Work out the finished part from the listing and answer in its coordinate system (mm). A direction names the side the tool comes from. Give positions to 0.01 mm unless a question says otherwise; leave off trailing zeros. Loops run counter-clockwise (first coordinate to the right, second up) from the corner with the lowest first, then second, coordinate; pieces in that order, holes last. Notation, with made-up numbers: (71.25, 34.25) - (122.25, 34.25) arc R31 cw to (122.25, 67.25) - close; hole circle Ø4 at (27.5, 13). An arc over 180 degrees is marked (long way). One line per item, written item: value.
from build123d import *

# Parameters (mm, degrees)
F1_DEPTH  = 15
F4_DEPTH  = 80
F6_DEPTH  = 80
F7_DEPTH  = 80
F9_DEPTH  = 30
F11_D     = 15
F11_DEPTH = 80
F11_TIP   = 4.5064546427
F14_D     = 15
F14_DEPTH = 80
F14_TIP   = 4.5064546427
F15_D     = 15
F15_DEPTH = 80
F15_TIP   = 4.5064546427


with BuildPart() as f1:
    # F0 (on Top) → F1 (new body)
    with BuildSketch(Plane.XY):
        Polygon((-20, 0), (0, 0), (20, 0), (40, 34.6410161514), (20, 69.2820323028), (0, 69.2820323028), (-20, 69.2820323028), (-40, 34.6410161514), align=None)
    extrude(amount=-F1_DEPTH)

    # F3 (on face) → F4 (cut)
    with BuildSketch(Plane(origin=(-45, 25.9807621135, 0), x_dir=(-0.5, -0.8660254038, 0), z_dir=(-0.8660254038, 0.5, 0))):
        with BuildLine():
            ThreePointArc((-25, -12.5), (-20, -7.5), (-25, -2.5))
            Line((-25, -2.5), (-35, -2.5))
            ThreePointArc((-35, -2.5), (-40, -7.5), (-35, -12.5))
            Line((-35, -12.5), (-25, -12.5))
        make_face()
    extrude(amount=-F4_DEPTH, mode=Mode.SUBTRACT)

    # F5 (on face) → F6 (cut)
    with BuildSketch(Plane.XZ):
        with BuildLine():
            ThreePointArc((5, -12.5), (10, -7.5), (5, -2.5))
            Line((5, -2.5), (-5, -2.5))
            ThreePointArc((-5, -2.5), (-10, -7.5), (-5, -12.5))
            Line((-5, -12.5), (5, -12.5))
        make_face()
    extrude(amount=-F6_DEPTH, mode=Mode.SUBTRACT)

    # F2 (on face) → F7 (cut)
    with BuildSketch(Plane(origin=(-15, -8.6602540378, 0), x_dir=(0.5, -0.8660254038, 0), z_dir=(-0.8660254038, -0.5, 0))):
        with BuildLine():
            ThreePointArc((-35, -2.5), (-40, -7.5), (-35, -12.5))
            Line((-35, -12.5), (-25, -12.5))
            ThreePointArc((-25, -12.5), (-20, -7.5), (-25, -2.5))
            Line((-25, -2.5), (-35, -2.5))
        make_face()
    extrude(amount=-F7_DEPTH, mode=Mode.SUBTRACT)

    # F8 (on face) → F9 (join)
    with BuildSketch(Plane.XY):
        Polygon((11.5, 54.5596004384), (-11.5, 54.5596004384), (-23, 34.6410161514), (-11.5, 14.7224318643), (11.5, 14.7224318643), (23, 34.6410161514), align=None)
    extrude(amount=F9_DEPTH)

    # F11
    with Locations(Plane.XZ.offset(-14.7224318643)):
        with Locations((0, 15)):
            Hole(F11_D / 2, depth=F11_DEPTH)
            with Locations((0, 0, -(F11_DEPTH + F11_TIP / 2))):  # 118° drill point
                Cone(0, F11_D / 2, F11_TIP, mode=Mode.SUBTRACT)

    # F14
    with Locations(Plane(origin=(-2.25, -1.2990381057, 0), x_dir=(0.5, -0.8660254038, 0), z_dir=(-0.8660254038, -0.5, 0))):
        with Locations((-30, 15)):
            Hole(F14_D / 2, depth=F14_DEPTH)
            with Locations((0, 0, -(F14_DEPTH + F14_TIP / 2))):  # 118° drill point
                Cone(0, F14_D / 2, F14_TIP, mode=Mode.SUBTRACT)

    # F15
    with Locations(Plane(origin=(-32.25, 18.6195461814, 0), x_dir=(-0.5, -0.8660254038, 0), z_dir=(-0.8660254038, 0.5, 0))):
        with Locations((-30, 15)):
            Hole(F15_D / 2, depth=F15_DEPTH)
            with Locations((0, 0, -(F15_DEPTH + F15_TIP / 2))):  # 118° drill point
                Cone(0, F15_D / 2, F15_TIP, mode=Mode.SUBTRACT)


solid = f1.part
1. For faces 1 (the flat face through (-13.336, 51.379, 14.79)), 2 (the flat face through (21.164, 37.821, 14.79)), 3 (the cylindrical face through (-10, 9.9, -7.4)), 4 (the cylindrical face through (-26.41, 30.94, -7.39)), determine the directions among +Z, -Z, +X, -X, +Y, -Y from which every point of the face is accessible in a straight line to the end or side of a thin tool.
Output:
face 1: +Z, -X, +Y
face 2: +Z, +X, +Y
face 3: +Y, -Y
face 4: none
2. Find the intervals of material crossed by line 1 along Z through (x, y) = (0, 47.5); line 2 along Z through (x, y) = (-21.5, 23); line 3 along Y through (x, z) = (12, 21), in increasing order.
Output:
line 1: z = -15 to -12.5, -2.5 to 7.5, 22.5 to 30
line 2: z = -15 to -12.5, -2.5 to 0
line 3: y = 15.59 to 22.52, 32.91 to 36.37, 46.77 to 53.69
3. The mould has two halves that part along Z. Classify faces 5 (the flat face through (0, 35, 30)), 6 (the flat face through (13.336, 17.903, 14.79)), 7 (the cylindrical face through (-12.826, 40.919, 22.436)): released by +Z, released by -Z, zero draft, split by the parting line, or undercut.
Output:
face 5: released by +Z
face 6: zero draft
face 7: undercut
4. Section A-A (z = 18.5) is taken. Write down the section's boundary in (x, y).
Output:
outline: (-23, 34.64) - (-20.57, 30.43) - (-13.27, 34.64) - (-20.57, 38.86) - close; (-13.93, 18.94) - (-11.5, 14.72) - (-6.63, 14.72) - (-6.63, 23.15) - close; (-13.93, 50.34) - (-6.63, 46.13) - (-6.63, 54.56) - (-11.5, 54.56) - close; (6.63, 14.72) - (11.5, 14.72) - (13.93, 18.94) - (6.63, 23.15) - close; (6.63, 46.13) - (13.93, 50.34) - (11.5, 54.56) - (6.63, 54.56) - close; (13.27, 34.64) - (20.57, 30.43) - (23, 34.64) - (20.57, 38.86) - close
5. Section D-D (z = -7.5) is taken. Write down the section's boundary in (x, y), and give its area (3 significant figures).
Output:
outline: (-40, 34.64) - (-35, 25.98) - (-20, 34.64) - (-35, 43.3) - close; (-25, 8.66) - (-20, 0) - (-10, 0) - (-10, 17.32) - close; (-25, 60.62) - (-10, 51.96) - (-10, 69.28) - (-20, 69.28) - close; (10, 0) - (20, 0) - (25, 8.66) - (10, 17.32) - close; (10, 51.96) - (25, 60.62) - (20, 69.28) - (10, 69.28) - close; (20, 34.64) - (35, 25.98) - (40, 34.64) - (35, 43.3) - close
area: 1,040 mm²
6. Flat-ended cylindrical pins translate along their axes: pin 1 Ø3 at (y, z) = (24.5, 5) entering from +X; pin 2 Ø1.5 at (y, z) = (36.5, 7.5) entering from +X; pin 3 Ø10 at (x, z) = (20.5, 1) entering from -Y; pin 4 Ø11.5 at (x, z) = (5.5, 13.5) entering from -Y. Find the tip coordinate at first contact, or state that the pin passes through.
Output:
pin 1: stops at x = 18.01
pin 2: stops at x = 22.36
pin 3: stops at y = 0
pin 4: stops at y = 14.72
7. Section C-C (y = 39) is taken. Count the separate pieces of the cut face and the enclosed holes in it, and give its area (3 significant figures).
Output:
separate pieces: 2
enclosed holes: 1
area: 1,290 mm²
8. Section B-B (y = 7.5) is taken. Write down the section's boundary in (x, z), and give its area (3 significant figures).
Output:
outline: (-24.33, -15) - (24.33, -15) - (24.33, 0) - (-24.33, 0) - close; hole (-5, -12.5) - (5, -12.5) arc R5 ccw to (5, -2.5) - (-5, -2.5) arc R5 ccw to start
area: 551 mm²
